from build123d import *

# Parameters (mm, degrees)
SKETCH1_W           = 304.8
SKETCH1_H           = 152.4
BOSS_EXTRUDE1_DEPTH = 12.7
SKETCH2_W           = 38.1
SKETCH2_H           = 50.8
BOSS_EXTRUDE2_DEPTH = 76.2
SKETCH3_W           = 101.6
SKETCH3_H           = 101.6
BOSS_EXTRUDE3_DEPTH = 50.8


with BuildPart() as part:
    # Sketch1 → Boss-Extrude1 (new body)
    with BuildSketch(Plane(origin=(0, 0, 0), x_dir=(1, 0, 0), z_dir=(0, 1, 0))):
        Rectangle(SKETCH1_W, SKETCH1_H)
    extrude(amount=BOSS_EXTRUDE1_DEPTH)

    # Sketch2 → Boss-Extrude2 (add)
    with BuildSketch(Plane(origin=(0, 12.7, 0), x_dir=(1, 0, 0), z_dir=(0, 1, 0))):
        with Locations((133.070932654, 3.267194716)):
            Rectangle(SKETCH2_W, SKETCH2_H)
    extrude(amount=BOSS_EXTRUDE2_DEPTH)

    # Sketch3 → Boss-Extrude3 (add)
    with BuildSketch(Plane(origin=(0, 12.7, 0), x_dir=(1, 0, 0), z_dir=(0, 1, 0))):
        with Locations((-101.6, 0.217888901)):
            Rectangle(SKETCH3_W, SKETCH3_H)
    extrude(amount=BOSS_EXTRUDE3_DEPTH)


solid = part.part
Design review of the part built by this model. Coordinates are the model's own, in mm. A direction names the side the tool comes from. Give positions to 0.01 mm unless a question says otherwise; leave off trailing zeros. Write each loop counter-clockwise with the first axis right and the second up, starting at its lowest first coordinate (ties: lowest second). Pieces come first, ordered by that corner, then holes. Notation, with made-up numbers: M 8,-32 L 37,-32 A26 cw 37,-13 Z; hole C 38,66 d10. An arc over 180 degrees is marked long. Return JSON: item names as keys, results as strings. Group by question number.
Item 1: Take a section at C-C (x = -87.5). Give the boundary of the cut face in (y, z).
Item 2: Take a section at A-A (y = 43). Give the boundary of the cut face in (x, z), plus the area to 3 significant figures.
Item 3: Clearance check with flat-ended pins moving along their axes: pin 1 Ø15 at (x, y) = (-94.5, 47.5) entering from +Z; pin 2 Ø1 at (x, z) = (-68.5, 27.5) entering from +Y; pin 3 Ø12 at (y, z) = (36.5, -23) entering from +X. State where each tip first meets the part, or that it passes through.
Item 4: Take a section at B-B (z = -11.5). Give the boundary of the cut face in (x, y).
Item 5: Take a section at D-D (y = 69). Give the boundary of the cut face in (x, z).
Item 6: Tool access review of faces 5 (the flat face through (114.021, 50, -3)), 6 (the flat face through (-102, 38, -51.018)), 7 (the flat face through (152.121, 50, -3)): name each direction out of +Z, -Z, +X, -X, +Y, -Y from which nothing blocks a thin tool from reaching the whole face with its end or side.
Item 7: The part is to be moulded in two halves that separate along X. For faces 1 (the flat face through (-50.8, 38, 0)), 2 (the flat face through (32, 12.7, -1)), 3 (the flat face through (152.4, 6, 1)), 4 (the flat face through (133, 50, -28.667)), say which applies: pulls with the +X half, pulls with the -X half, needs draft (parallel to the pull), parting line crosses it, or undercut.
Item 8: Wall thickness on line 1 along X through (y, z) = (60.5, 3); line 2 along Z through (x, y) = (128.5, 53); line 3 along Y through (x, z) = (-65, -25.5): over which ranges is each line inside the solid? List them lowest first.
Return value:
{
 "1": {"outline": "M 0,-76.2 L 12.7,-76.2 L 12.7,-51.02 L 63.5,-51.02 L 63.5,50.58 L 12.7,50.58 L 12.7,76.2 L 0,76.2 Z"},
 "2": {"outline": "M -152.4,-51.02 L -50.8,-51.02 L -50.8,50.58 L -152.4,50.58 Z; M 114.02,-28.67 L 152.12,-28.67 L 152.12,22.13 L 114.02,22.13 Z", "area": "12,300 mm2"},
 "3": {"pin 1": "stops at z = 50.58", "pin 2": "stops at y = 63.5", "pin 3": "stops at x = 152.12"},
 "4": {"outline": "M -152.4,0 L 152.4,0 L 152.4,12.7 L 152.12,12.7 L 152.12,88.9 L 114.02,88.9 L 114.02,12.7 L -50.8,12.7 L -50.8,63.5 L -152.4,63.5 Z"},
 "5": {"outline": "M 114.02,-28.67 L 152.12,-28.67 L 152.12,22.13 L 114.02,22.13 Z"},
 "6": {"face 5": "+Z, -Z, +Y", "face 6": "-Z, +X, -X, +Y", "face 7": "+Z, -Z, +X, +Y"},
 "7": {"face 1": "undercut", "face 2": "undercut", "face 3": "pulls with the +X half", "face 4": "needs draft"},
 "8": {"line 1": "x = -152.4 to -50.8, 114.02 to 152.12", "line 2": "z = -28.67 to 22.13", "line 3": "y = 0 to 63.5"}
}
